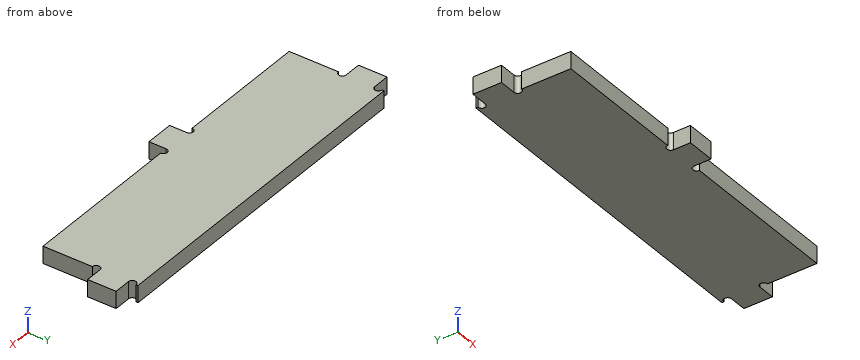
Autodesk Inventor part; units mm, degrees
ref_plane "YZ Plane" through (0, 0, 0) normal (1, 0, 0) x (0, 1, 0)
ref_plane "XZ Plane" through (0, 0, 0) normal (0, 1, 0) x (-1, 0, 0)
ref_plane "XY Plane" through (0, 0, 0) normal (0, 0, 1) x (1, 0, 0)
sketch "CONTOURS" plane through (0, 0, 0) normal (0, 0, 1) x (1, 0, 0)
  arc A0 (113.8436, 518.7397) -> (113.8436, 526.7397) centre (113.8436, 522.7397) ccw
  line L0 (113.8436, 526.7397) -> (113.8436, 528.7397)
  line L1 (113.8436, 528.7397) -> (472.3436, 528.7397)
  line L2 (472.3436, 528.7397) -> (472.3436, 526.7397)
  arc A1 (472.3436, 526.7397) -> (472.3436, 518.7397) centre (472.3436, 522.7397) ccw
  line L3 (472.3436, 518.7397) -> (490.3436, 518.7397)
  line L4 (490.3436, 518.7397) -> (490.3436, 488.7397)
  line L5 (490.3436, 488.7397) -> (472.3436, 488.7397)
  arc A2 (472.3436, 488.7397) -> (472.3436, 480.7397) centre (472.3436, 484.7397) ccw
  line L6 (472.3436, 480.7397) -> (472.3436, 428.7397)
  line L7 (472.3436, 428.7397) -> (301.0936, 428.7397)
  arc A3 (301.0936, 428.7397) -> (293.0936, 428.7397) centre (297.0936, 428.7397) ccw
  line L8 (293.0936, 428.7397) -> (293.0936, 410.7397)
  line L9 (293.0936, 410.7397) -> (263.0936, 410.7397)
  line L10 (263.0936, 410.7397) -> (263.0936, 428.7397)
  arc A4 (263.0936, 428.7397) -> (255.0936, 428.7397) centre (259.0936, 428.7397) ccw
  line L11 (255.0936, 428.7397) -> (113.8436, 428.7397)
  line L12 (113.8436, 428.7397) -> (113.8436, 480.7397)
  arc A5 (113.8436, 480.7397) -> (113.8436, 488.7397) centre (113.8436, 484.7397) ccw
  line L13 (113.8436, 488.7397) -> (95.8436, 488.7397)
  line L14 (95.8436, 488.7397) -> (95.8436, 518.7397)
  line L15 (95.8436, 518.7397) -> (113.8436, 518.7397)
extrude "Extrusion1" add sketch "CONTOURS" along normal blind 18
properties part number "Layer 1 Plank" material "Wood (Birch)"
The model under review builds one solid part; all positions refer to its coordinate system, in mm. Coordinates: 2 decimals unless noted, no trailing zeros. Loops run counter-clockwise (first coordinate to the right, second up) from the corner with the lowest first, then second, coordinate; pieces in that order, holes last. Notation, with made-up numbers: (43, 66.25) -> (70, 66.25) arc R19 ccw to (70, 103.25) -> close; hole circle Ø4 at (87.5, 5). An arc over 180 degrees is marked (long way). Answer as CSV lines item,"result".
Item 1: Insertion check: pin 1 (1.5 mm diameter, centred on x = 371, y = 455.5, fed in from -Z); pin 2 (0.6 mm diameter, centred on y = 527.5, z = 13, fed in from +X); pin 3 (5.5 mm diameter, centred on y = 460.5, z = 8, fed in from -X); pin 4 (5.5 mm diameter, centred on x = 357.5, z = 11, fed in from -Y). Each pin has a flat end and moves straight along its axis. Give the tip position at first contact, or say it passes through.
Results below:
pin 1,"stops at z = 0"
pin 2,"stops at x = 472.34"
pin 3,"stops at x = 113.84"
pin 4,"stops at y = 428.74"
Item 2: Take a section at A-A, the plane z = 7.5. State the section outline as (x, y) points.
Results below:
outline,"(95.84, 488.74) -> (113.84, 488.74) arc R4 cw to (113.84, 480.74) -> (113.84, 428.74) -> (255.09, 428.74) arc R4 cw to (263.09, 428.74) -> (263.09, 410.74) -> (293.09, 410.74) -> (293.09, 428.74) arc R4 cw to (301.09, 428.74) -> (472.34, 428.74) -> (472.34, 480.74) arc R4 cw to (472.34, 488.74) -> (490.34, 488.74) -> (490.34, 518.74) -> (472.34, 518.74) arc R4 cw to (472.34, 526.74) -> (472.34, 528.74) -> (113.84, 528.74) -> (113.84, 526.74) arc R4 cw to (113.84, 518.74) -> (95.84, 518.74) -> close"
Item 3: Take a section at C-C, the plane y = 437.5. State the section outline as (x, z) points.
Results below:
outline,"(113.84, 0) -> (472.34, 0) -> (472.34, 18) -> (113.84, 18) -> close"
Item 4: For L1, parallel to X at y = 429, z = 2.5; L2, parallel to Y at x = 459, z = 2.5; L3, parallel to X at y = 477, z = 15.25, list the stretches that pass through material, from the lowest coordinate up.
Results below:
L1,"x = 113.84 to 255.1, 263.09 to 293.1, 301.09 to 472.34"
L2,"y = 428.74 to 528.74"
L3,"x = 113.84 to 472.34"
Item 5: Take a section at B-B, the plane x = 218. State the section outline as (y, z) points.
Results below:
outline,"(428.74, 0) -> (528.74, 0) -> (528.74, 18) -> (428.74, 18) -> close"
